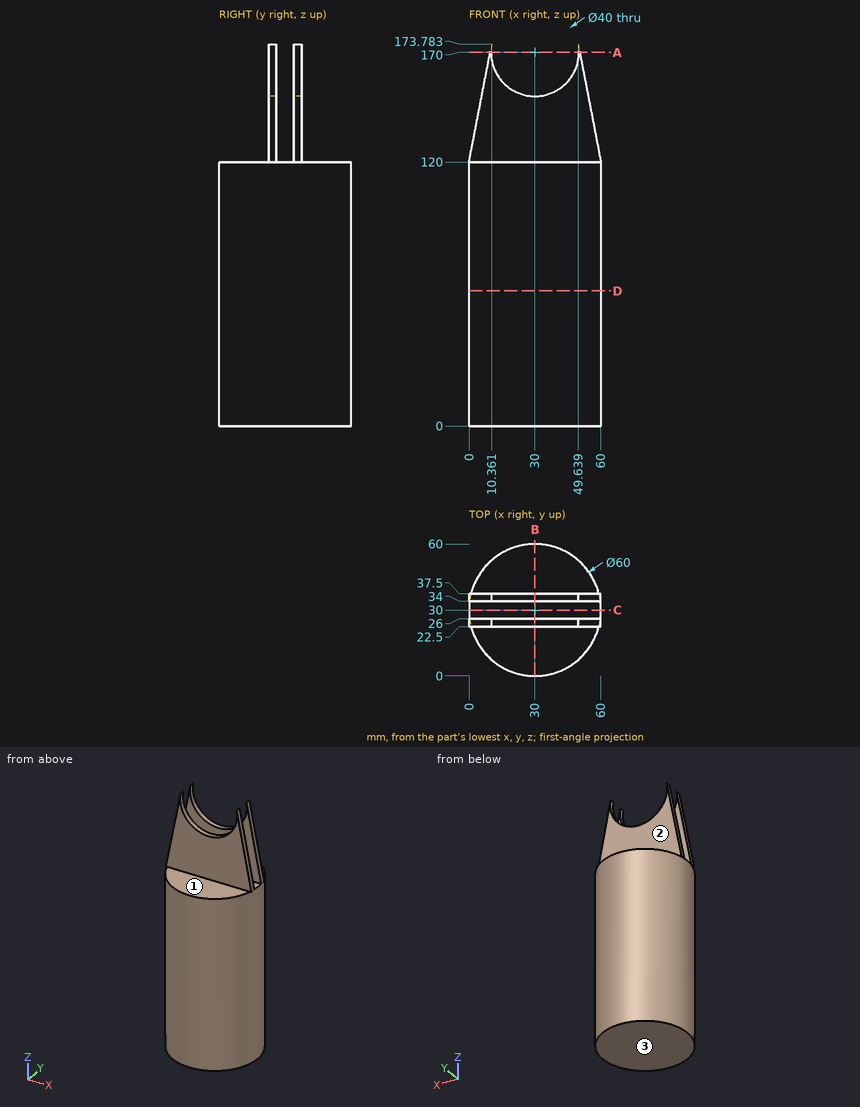
For this review, use the dimensioned drawing (mm, ordinates from the lowest corner) and the shaded views. A direction names the side the tool comes from. Give positions to 0.01 mm unless a question says otherwise; leave off trailing zeros. Loops run counter-clockwise (first coordinate to the right, second up) from the corner with the lowest first, then second, coordinate; pieces in that order, holes last.
Item 1: For line 1 along Y through (x, z) = (22, 142.5); line 2 along X through (y, z) = (25, 170); line 3 along Z through (x, y) = (41.5, 30), list the stretches that pass through material, from the lowest coordinate up.
Item 2: Take a section at B-B, the plane x = 30. State the section outline as (y, z) points, and give its area (3 significant figures).
Item 3: Take a section at C-C, the plane y = 30. State the section outline as (x, z) points.
Item 4: Tool access review of the marked faces 1, 2 and 3: name each direction out of +Z, -Z, +X, -X, +Y, -Y from which nothing blocks a thin tool from reaching the whole face with its end or side.
Item 5: Insertion check: pin 1 (3 mm diameter, centred on y = 38, z = 34, fed in from -X); pin 2 (18 mm diameter, centred on x = 27.5, y = 16, fed in from +Z); pin 3 (2.5 mm diameter, centred on x = 18, y = 29, fed in from +Z). Each pin has a flat end and moves straight along its axis. Give the tip position at first contact, or say it passes through.
Item 6: Take a section at D-D, the plane z = 61.5. State the section outline as (x, y) points, and give its area (3 significant figures).
Item 7: Take a section at A-A, the plane z = 170. State the section outline as (x, y) points.
Calculated:
1. line 1: y = 22.5 to 26, 34 to 37.5
1. line 2: x = 9.63 to 10, 50 to 50.37
1. line 3: z = 0 to 120
2. outline: (0, 0) - (60, 0) - (60, 120) - (37.5, 120) - (37.5, 150) - (34, 150) - (34, 120) - (26, 120) - (26, 150) - (22.5, 150) - (22.5, 120) - (0, 120) - close
2. area: 7,410 mm2
3. outline: (0, 0) - (60, 0) - (60, 120) - (0, 120) - close
4. face 1: +Z, +X, -X, -Y
4. face 2: +Z, +X, -X, +Y
4. face 3: -Z, +X, -X, +Y, -Y
5. pin 1: stops at x = 0.71
5. pin 2: stops at z = 152
5. pin 3: stops at z = 120
6. outline: circle Ø60 at (30, 30)
6. area: 2,830 mm2
7. outline: (9.63, 22.5) - (10, 22.5) - (10, 26) - (9.63, 26) - close; (9.63, 34) - (10, 34) - (10, 37.5) - (9.63, 37.5) - close; (50, 22.5) - (50.37, 22.5) - (50.37, 26) - (50, 26) - close; (50, 34) - (50.37, 34) - (50.37, 37.5) - (50, 37.5) - close
